```python
from build123d import *

# Parameters (mm, degrees)
SM_BASE_FLANGE_1_DEPTH = 48
SKETCH_6_R             = 2
CUT_EXTRUDE_1_DEPTH    = 10
SKETCH_7_R             = 13
SKETCH_7_R_2           = 2
CUT_EXTRUDE_2_DEPTH    = 10
CHAMFER_1_SIZE         = 10
EXTRUDE_START          = -2
EXTRUDE_1_DEPTH        = 2


# Sheet-metal steps are written as plain solids
with BuildPart() as part:
    # Sketch 1 → 基体-法兰1 (new body)
    with BuildSketch(Plane.XY):
        with BuildLine():
            Line((0, 50), (0, 4))
            ThreePointArc((0, 4), (1.171572875, 1.171572875), (4, 0))
            Line((4, 0), (47, 0))
            Line((47, 0), (47, 2))
            Line((47, 2), (4, 2))
            ThreePointArc((4, 2), (2.585786438, 2.585786438), (2, 4))
            Line((2, 4), (2, 50))
            Line((2, 50), (0, 50))
        make_face()
    extrude(amount=SM_BASE_FLANGE_1_DEPTH)

    # 草图6 → 切除-拉伸1 (cut)
    with BuildSketch(Plane(origin=(0, 2, 0), x_dir=(1, 0, 0), z_dir=(0, 1, 0))):
        with Locations(Location((38, -9, 0), (0, 0, 270))):
            Circle(SKETCH_6_R)
        with Locations(Location((38, -39, 0), (0, 0, 270))):
            Circle(SKETCH_6_R)
        with Locations(Location((16, -9, 0), (0, 0, 270))):
            Circle(SKETCH_6_R)
        with Locations(Location((16, -39, 0), (0, 0, 270))):
            Circle(SKETCH_6_R)
    extrude(amount=-CUT_EXTRUDE_1_DEPTH, mode=Mode.SUBTRACT)

    # 草图7 → 切除-拉伸2 (cut)
    with BuildSketch(Plane(origin=(2, 0, 0), x_dir=(0, 0, -1), z_dir=(1, 0, 0))):
        with Locations(Location((-21, 28, 0), (0, 0, 90))):
            Circle(SKETCH_7_R)
        with Locations(Location((-21, 45.5, 0), (0, 0, 90))):
            Circle(SKETCH_7_R_2)
        with Locations(Location((-3.5, 28, 0), (0, 0, 90))):
            Circle(SKETCH_7_R_2)
        with Locations(Location((-21, 10.5, 0), (0, 0, 90))):
            Circle(SKETCH_7_R_2)
        with Locations(Location((-38.5, 28, 0), (0, 0, 90))):
            Circle(SKETCH_7_R_2)
    extrude(amount=-CUT_EXTRUDE_2_DEPTH, mode=Mode.SUBTRACT)

    # 倒角1
    chamfer_1_edges = [part.edges().sort_by_distance(p)[0] for p in [
        (1, 50, 48),
        (1, 50, 0),
    ]]
    chamfer(chamfer_1_edges, length=CHAMFER_1_SIZE)

    # 草图8 → 凸台-拉伸1 (add)
    with BuildSketch(Plane.XY.offset(48).offset(EXTRUDE_START)):
        with BuildLine():
            Line((2, 22), (22, 2))
            Line((22, 2), (4, 2))
            ThreePointArc((4, 2), (2.585786438, 2.585786438), (2, 4))
            Line((2, 4), (2, 22))
        make_face()
    extrude_1 = extrude(amount=EXTRUDE_1_DEPTH)

    # 镜向1: 凸台-拉伸1 across plane
    add(extrude_1.mirror(Plane.XY.offset(24)))


solid = part.part
```
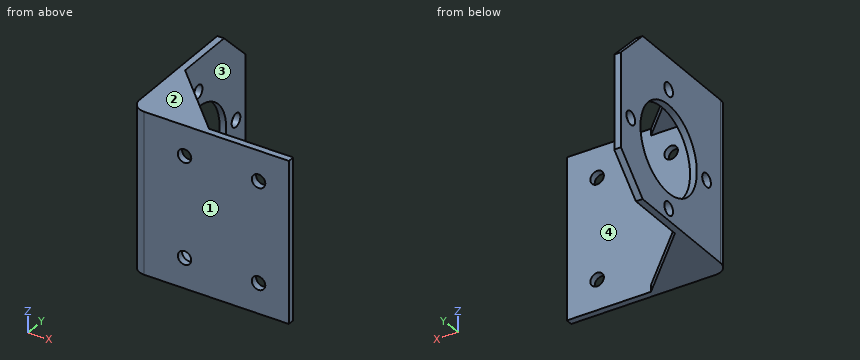
Work out the finished part from the listing and answer in its coordinate system (mm). Face numbers are marked on the shaded views. Give positions to 0.01 mm unless a question says otherwise; leave off trailing zeros. Write each loop counter-clockwise with the first axis right and the second up, starting at its lowest first coordinate (ties: lowest second). Pieces come first, ordered by that corner, then holes. Notation, with made-up numbers: (35, 33.25) -> (47, 33.25) arc R26 ccw to (47, 49.25) -> close; hole circle Ø6 at (53.25, -23). An arc over 180 degrees is marked (long way). Write item = value, one per line.
Q1. Section D-D on y = 28 is taken. Determine the outline of the cut face in (x, z), and give its area (3 significant figures).
Computed values:
outline = (0, 0) -> (2, 0) -> (2, 1.5) -> (0, 1.5) -> close; (0, 5.5) -> (2, 5.5) -> (2, 8) -> (0, 8) -> close; (0, 34) -> (2, 34) -> (2, 36.5) -> (0, 36.5) -> close; (0, 40.5) -> (2, 40.5) -> (2, 48) -> (0, 48) -> close
area = 28.0 mm^2
Q2. Section C-C on z = 33 is taken. Determine the outline of the cut face in (x, y), and give its area (3 significant figures).
Computed values:
outline = (0, 4) arc R4 ccw to (4, 0) -> (47, 0) -> (47, 2) -> (4, 2) arc R2 cw to (2, 4) -> (2, 23) -> (0, 23) -> close; (0, 33) -> (2, 33) -> (2, 50) -> (0, 50) -> close
area = 167 mm^2
Q3. Section A-A on x = 38 is taken. Determine the outline of the cut face in (y, z).
Computed values:
outline = (0, 0) -> (2, 0) -> (2, 7) -> (0, 7) -> close; (0, 11) -> (2, 11) -> (2, 37) -> (0, 37) -> close; (0, 41) -> (2, 41) -> (2, 48) -> (0, 48) -> close
Q4. Flat-ended cylindrical pins translate along their axes: pin 1 Ø23 at (y, z) = (26.5, 35) entering from +X; pin 2 Ø2.5 at (x, z) = (38, 9) entering from +Y; pin 3 Ø2 at (x, z) = (6.5, 30) entering from +Y. Find the tip coordinate at first contact, or state that the pin passes through.
Computed values:
pin_1 = 2
pin_2 = through
pin_3 = 2
Q5. Consider line 1 along Z through (x, y) = (1.5, 28); line 2 along X through (y, z) = (1.05, 39); line 3 along Z through (x, y) = (0.65, 10.5). Determine where each line is inside the solid, lowest interval first.
Computed values:
line_1 = 0 to 1.5, 5.5 to 8, 34 to 36.5, 40.5 to 48
line_2 = 1.3 to 14, 18 to 36, 40 to 47
line_3 = 0 to 19, 23 to 48
Q6. Section B-B on y = 10.5 is taken. Determine the outline of the cut face in (x, z), and give its area (3 significant figures).
Computed values:
outline = (0, 0) -> (13.5, 0) -> (13.5, 2) -> (2, 2) -> (2, 19) -> (0, 19) -> close; (0, 23) -> (2, 23) -> (2, 46) -> (13.5, 46) -> (13.5, 48) -> (0, 48) -> close
area = 134 mm^2
Q7. For a pull along Z with two mould halves and no side action, classify the marked faces 1, 2, 3 and 4 as pulls with the +Z half, pulls with the -Z half, needs draft (parallel to the pull), parting line crosses it, or undercut.
Computed values:
face_1 = needs draft
face_2 = pulls with the +Z half
face_3 = undercut
face_4 = undercut
